```python
from build123d import *

# Parameters (mm, degrees)
BOSS_EXTRUDE2_DEPTH = 30
FILLET1_R           = 5
CUT_EXTRUDE1_REACH  = 6
SKETCH6_R           = 1.5
SKETCH6_3_R         = 2.5
CUT_EXTRUDE2_DEPTH  = 2
CUT_EXTRUDE3_REACH  = 8
SKETCH8_R           = 1.5


with BuildPart() as part:
    # Sketch3 → Boss-Extrude2 (new body)
    with BuildSketch(Plane(origin=(0, 0, 0), x_dir=(0, 0, -1), z_dir=(1, 0, 0))):
        with BuildLine():
            Line((0, 15), (0, -15))
            ThreePointArc((0, -15), (-1.757359313, -19.242640687), (-6, -21))
            Line((-6, -21), (-24, -21))
            Line((-24, -21), (-24, -25))
            Line((-24, -25), (-4, -25))
            ThreePointArc((-4, -25), (3.071067812, -22.071067812), (6, -15))
            Line((6, -15), (6, 15))
            Line((6, 15), (0, 15))
        make_face()
    extrude(amount=BOSS_EXTRUDE2_DEPTH)

    # Fillet1
    fillet1_edges = [part.edges().sort_by_distance(p)[0] for p in [
        (0, 15, -3),
        (30, -23, 24),
        (30, 15, -3),
        (0, -23, 24),
    ]]
    fillet(fillet1_edges, radius=FILLET1_R)

    # Sketch6 → Cut-Extrude1 (cut, up to next)
    with BuildSketch(Plane(origin=(0, -21, 0), x_dir=(1, 0, 0), z_dir=(0, 1, 0)), mode=Mode.PRIVATE) as cut_extrude1_sk1:
        with Locations((8, -18)):
            Circle(SKETCH6_R)
    cut_extrude1_tool1 = extrude(cut_extrude1_sk1.sketch, amount=-CUT_EXTRUDE1_REACH, mode=Mode.PRIVATE) & part.part
    add(cut_extrude1_tool1.solids().sort_by_distance((8, -21, 18))[0], mode=Mode.SUBTRACT)
    # Sketch6 → Cut-Extrude1 (cut, up to next)
    with BuildSketch(Plane(origin=(0, -21, 0), x_dir=(1, 0, 0), z_dir=(0, 1, 0)), mode=Mode.PRIVATE) as cut_extrude1_sk2:
        with Locations((22, -18)):
            Circle(SKETCH6_R)
    cut_extrude1_tool2 = extrude(cut_extrude1_sk2.sketch, amount=-CUT_EXTRUDE1_REACH, mode=Mode.PRIVATE) & part.part
    add(cut_extrude1_tool2.solids().sort_by_distance((22, -21, 18))[0], mode=Mode.SUBTRACT)

    # Sketch6_3 → Cut-Extrude2 (cut)
    with BuildSketch(Plane(origin=(0, -21, 0), x_dir=(1, 0, 0), z_dir=(0, 1, 0))):
        with Locations((8, -18)):
            Circle(SKETCH6_3_R)
        with Locations((22, -18)):
            Circle(SKETCH6_3_R)
    extrude(amount=-CUT_EXTRUDE2_DEPTH, mode=Mode.SUBTRACT)

    # Sketch8 → Cut-Extrude3 (cut, up to next)
    with BuildSketch(Plane.XY, mode=Mode.PRIVATE) as cut_extrude3_sk1:
        with Locations((8, 5)):
            Circle(SKETCH8_R)
    cut_extrude3_tool1 = extrude(cut_extrude3_sk1.sketch, amount=-CUT_EXTRUDE3_REACH, mode=Mode.PRIVATE) & part.part
    add(cut_extrude3_tool1.solids().sort_by_distance((8, 5, 0))[0], mode=Mode.SUBTRACT)
    # Sketch8 → Cut-Extrude3 (cut, up to next)
    with BuildSketch(Plane.XY, mode=Mode.PRIVATE) as cut_extrude3_sk2:
        with Locations((22, 5)):
            Circle(SKETCH8_R)
    cut_extrude3_tool2 = extrude(cut_extrude3_sk2.sketch, amount=-CUT_EXTRUDE3_REACH, mode=Mode.PRIVATE) & part.part
    add(cut_extrude3_tool2.solids().sort_by_distance((22, 5, 0))[0], mode=Mode.SUBTRACT)


solid = part.part
```
Geometry check sheet. Reference: the model listing, model coordinates, mm. A direction names the side the tool comes from. Give positions to 0.01 mm unless a question says otherwise; leave off trailing zeros. Write each loop counter-clockwise with the first axis right and the second up, starting at its lowest first coordinate (ties: lowest second). Pieces come first, ordered by that corner, then holes. Notation, with made-up numbers: (-32.5, 63) -> (22.5, 63) arc R15 ccw to (22.5, 79) -> close; hole circle Ø6 at (21.5, 35.5). An arc over 180 degrees is marked (long way). Use one line per item in the form item = value.
Item 1: Sectioned sample at B-B on z = 18. Enter the section's corners in (x, y), plus the area to 3 significant figures.
Results list:
outline = (0, -25) -> (6.5, -25) -> (6.5, -23) -> (5.5, -23) -> (5.5, -21) -> (0, -21) -> close; (9.5, -25) -> (20.5, -25) -> (20.5, -23) -> (19.5, -23) -> (19.5, -21) -> (10.5, -21) -> (10.5, -23) -> (9.5, -23) -> close; (23.5, -25) -> (30, -25) -> (30, -21) -> (24.5, -21) -> (24.5, -23) -> (23.5, -23) -> close
area = 88.0 mm2
Item 2: Depth check by flat-ended pin: pin 1 Ø4 at (x, z) = (7, 19) entering from -Y; pin 2 Ø2.5 at (x, y) = (22, 5) entering from -Z; pin 3 Ø2 at (x, y) = (18.5, -18.5) entering from -Z; pin 4 Ø2 at (x, z) = (10.5, 14) entering from +Y. Enter the tip coordinate at first touch or a pass-through.
Results list:
pin_1 = -25
pin_2 = through
pin_3 = -5.68
pin_4 = -21
Item 3: Scan lines: line 1 (X direction, y = -21.6, z = 18); line 2 (X direction, y = -24.4, z = 18); line 3 (Y direction, x = 3, z = 15.25). Record each from-to range of solid material in increasing order.
Results list:
line_1 = 0 to 5.5, 10.5 to 19.5, 24.5 to 30
line_2 = 0 to 6.5, 9.5 to 20.5, 23.5 to 30
line_3 = -25 to -21
Item 4: Sectioned sample at D-D on z = -3.75. Enter the section's corners in (x, y).
Results list:
outline = (0, -21.32) -> (30, -21.32) -> (30, 10) arc R5 ccw to (25, 15) -> (5, 15) arc R5 ccw to (0, 10) -> close; hole circle Ø3 at (8, 5); hole circle Ø3 at (22, 5)
Item 5: Sectioned sample at C-C on y = 5. Enter the section's corners in (x, z).
Results list:
outline = (0, -6) -> (6.5, -6) -> (6.5, 0) -> (0, 0) -> close; (9.5, -6) -> (20.5, -6) -> (20.5, 0) -> (9.5, 0) -> close; (23.5, -6) -> (30, -6) -> (30, 0) -> (23.5, 0) -> close
Item 6: Mould release check, pull along Y, two halves, no side actions. Record for faces 1 (the cylindrical face through (6.8, 4.1, -3)), 2 (the cylindrical face through (28, -23, 23)), 3 (the flat face through (15, -25, 14)): released by +Y, released by -Y, zero draft, split by the parting line, or undercut.
Results list:
face_1 = undercut
face_2 = zero draft
face_3 = released by -Y
Item 7: Access from +Z, -Z, +X, -X, +Y, -Y to the whole of each face (thin tool, end or side, straight path). Record for faces 4 (the cylindrical face through (6.89, -23.99, 16.99)), 5 (the flat face through (15, 0, 0)), 6 (the cylindrical face through (10.385, -21.986, 17.249)).
Results list:
face_4 = +Y, -Y
face_5 = +Z, +X, -X, +Y
face_6 = +Y
Item 8: Sectioned sample at A-A on x = 22. Enter the section's corners in (y, z).
Results list:
outline = (-25, 4) arc R10 ccw to (-15, -6) -> (3.5, -6) -> (3.5, 0) -> (-15, 0) arc R6 cw to (-21, 6) -> (-21, 15.5) -> (-23, 15.5) -> (-23, 16.5) -> (-25, 16.5) -> close; (-25, 19.5) -> (-23, 19.5) -> (-23, 20.5) -> (-21, 20.5) -> (-21, 24) -> (-25, 24) -> close; (6.5, -6) -> (15, -6) -> (15, 0) -> (6.5, 0) -> close
